CAD build for the part. Positions are in the model's coordinates, mm. A direction names the side the tool comes from. Give positions to 0.01 mm unless a question says otherwise; leave off trailing zeros. Write each loop counter-clockwise with the first axis right and the second up, starting at its lowest first coordinate (ties: lowest second). Pieces come first, ordered by that corner, then holes. Notation, with made-up numbers: (53.25, 12.5) - (95.25, 12.5) arc R29 cw to (95.25, 40.5) - close; hole circle Ø1 at (-4, 59). An arc over 180 degrees is marked (long way). Put each result on its own line as item: value. Start each with the question number.
1. Tool access for faces 1 (the flat face through (46, 9.525, 25)), 2 (the flat face through (29, 9, 7.515)), 3 (the flat face through (-25.03, 22.06, 14.06)): list every direction of +Z, -Z, +X, -X, +Y, -Y with a clear straight run to the whole face (end or side of a thin tool).
2. Cut at A-A on y = 50. List the corners of the cut face in (x, z).
3. Mould opens along Y. For faces 4 (the cylindrical face through (16.81, 30.01, 14.06)), 5 (the cylindrical face through (-21.068, 42.22, 9.623)), 6 (the cylindrical face through (25.477, 0.209, 3.705)), 7 (the cylindrical face through (-15.38, -15.73, 14.06)) say: +Y half, -Y half, draft (parallel to the pull), parting line (faces both ways), or undercut.
4. Drop flat-ended pins along their axis: pin 1 (1 mm diameter, centred on y = 18, z = 3.5, fed in from -X); pin 2 (11.5 mm diameter, centred on x = 46, y = 15, fed in from -Z); pin 3 (4 mm diameter, centred on y = 7, z = 16, fed in from +X); pin 4 (8.5 mm diameter, centred on x = 47, z = 25, fed in from +Y). Give the stop position or say it passes through.
5. Cut at D-D on y = -10.5. List the corners of the cut face in (x, z) (3 decimals), and give its area (3 significant figures).
6. Cut at C-C on x = 21. List the corners of the cut face in (y, z) (3 decimals), and give its area (3 significant figures).
7. Cut at B-B on z = 22. List the corners of the cut face in (x, y) (3 decimals), and give its area (3 significant figures).
8. Wall check: line 1 (Z direction, x = 35, y = 15) (3 decimals); line 2 (X direction, y = 44, z = 14.25); line 3 (Y direction, x = 0, z = 9.5) (1 decimal). Give the ranges that are in metal, low to high.
from build123d import *

# Parameters (mm, degrees)
SKETCH1_R           = 9.525
SKETCH1_R_2         = 7
BOSS_EXTRUDE1_DEPTH = 28.52
CUT_EXTRUDE10_START = -9
CUT_EXTRUDE10_DEPTH = 9
SKETCH5_W           = 38
SKETCH5_H           = 13.49
CUT_EXTRUDE11_DEPTH = 89.917885715
EXTRUDE_THIN4_DEPTH = 9
SKETCH9_W           = 9
SKETCH9_H           = 9
BOSS_EXTRUDE3_DEPTH = 20
SKETCH10_W          = 9
SKETCH10_H          = 10
CUT_EXTRUDE12_DEPTH = 85.459250319


with BuildPart() as part:
    # Sketch1 → Boss-Extrude1 (new body)
    with BuildSketch(Plane.XY):
        with BuildLine():
            Line((-22, 0), (-28.14403802, 44.745229643))
            ThreePointArc((-28.14403802, 44.745229643), (-16.381808273, 59.200012083), (-2.762561842, 46.47967755))
            ThreePointArc((-2.762561842, 46.47967755), (23.974569133, 26.563983764), (57, 22))
            Line((57, 22), (57, 9.525))
            Line((57, 9.525), (35, 9.525))
            ThreePointArc((35, 9.525), (25.475, 0), (35, -9.525))
            Line((35, -9.525), (57, -9.525))
            Line((57, -9.525), (57, -22))
            Line((57, -22), (0, -22))
            ThreePointArc((0, -22), (-15.556349186, -15.556349186), (-22, 0))
        make_face()
        Circle(SKETCH1_R, mode=Mode.SUBTRACT)
        with Locations((-15.512561842, 46.47967755)):
            Circle(SKETCH1_R_2, mode=Mode.SUBTRACT)
    extrude(amount=BOSS_EXTRUDE1_DEPTH)

    # Sketch2 → Cut-Extrude10 (cut)
    with BuildSketch(Plane.XY.offset(28.52).offset(CUT_EXTRUDE10_START)):
        with BuildLine():
            Line((-28.14403802, 44.745229643), (-26.227740449, 30.789395608))
            ThreePointArc((-26.227740449, 30.789395608), (-9.369633943, 28.50012147), (2.563298764, 40.626194538))
            Line((2.563298764, 40.626194538), (-2.762561842, 46.47967755))
            ThreePointArc((-2.762561842, 46.47967755), (-16.381808273, 59.200012083), (-28.14403802, 44.745229643))
        make_face()
    extrude(amount=CUT_EXTRUDE10_DEPTH, mode=Mode.SUBTRACT)

    # Sketch5 → Cut-Extrude11 (cut, through all)
    with BuildSketch(Plane(origin=(0, 40, 0), x_dir=(1, 0, 0), z_dir=(0, 1, 0))):
        with Locations((38, -14.26)):
            Rectangle(SKETCH5_W, SKETCH5_H)
    extrude(amount=-CUT_EXTRUDE11_DEPTH, mode=Mode.SUBTRACT)



with BuildPart() as body_2:
    # Sketch8 → Extrude-Thin4 (new body)
    with BuildSketch(Plane.XY.offset(28.52)):
        Polygon((2.563298764, 40.626194538), (-6.432243018, 40.342948992), (-6.746960292, 50.337995417), (2.248581491, 50.621240963), align=None)
    extrude(amount=-EXTRUDE_THIN4_DEPTH)


with BuildPart() as part_1:
    add(part.part)

    add(body_2.part)  # Boss-Extrude3 merges body 2
    # Sketch9 → Boss-Extrude3 (add)
    with BuildSketch(Plane(origin=(-1.590121568, 50.500370473, 0), x_dir=(0.9995046425001054, 0.0314717273236879, 0), z_dir=(-0.0314717273236879, 0.9995046425001055, 0))):
        with Locations((-0.659394469, -24.02)):
            Rectangle(SKETCH9_W, SKETCH9_H)
    extrude(amount=-BOSS_EXTRUDE3_DEPTH)

    # Sketch10 → Cut-Extrude12 (cut, through all)
    with BuildSketch(Plane(origin=(3.838703059, 0.12087049, 0), x_dir=(0, 0, -1), z_dir=(0.9995046425001055, 0.03147172732368791, 0))):
        with Locations((-24.02, 45.525398608)):
            Rectangle(SKETCH10_W, SKETCH10_H)
    extrude(amount=-CUT_EXTRUDE12_DEPTH, mode=Mode.SUBTRACT)


solid = part_1.part
Report:
1. face 1: +Z, -Z, +X
1. face 2: +X, +Y, -Y
1. face 3: +Z, -Z, -X, -Y
2. outline: (-27.77, 0) - (-21.56, 0) - (-21.56, 19.52) - (-27.77, 19.52) - close; (-9.46, 0) - (-3.26, 0) - (-3.26, 19.52) - (-9.46, 19.52) - close
3. face 4: +Y half
3. face 5: undercut
3. face 6: undercut
3. face 7: -Y half
4. pin 1: stops at x = -24.54
4. pin 2: stops at z = 0
4. pin 3: stops at x = 19
4. pin 4: stops at y = 21.89
5. outline: (-19.333, 0) - (57, 0) - (57, 7.515) - (19, 7.515) - (19, 21.005) - (57, 21.005) - (57, 28.52) - (-19.333, 28.52) - close
5. area: 1,660 mm²
6. outline: (-22, 0) - (27.867, 0) - (27.867, 7.515) - (-22, 7.515) - close; (-22, 21.005) - (27.867, 21.005) - (27.867, 28.52) - (-22, 28.52) - close
6. area: 750 mm²
7. outline: (-26.228, 30.789) - (-22, 0) arc R22 ccw to (0, -22) - (57, -22) - (57, -9.525) - (35, -9.525) arc R9.525 cw to (35, 9.525) - (57, 9.525) - (57, 22) arc R67 cw to (2.563, 40.626) - (-6.432, 40.343) - (-6.118, 30.348) - (-5.44, 30.369) arc R19 cw to start; hole circle Ø19.05 at (0, 0)
7. area: 3,100 mm²
8. line 1: z = 0 to 7.515, 21.005 to 28.52
8. line 2: x = -28.04 to -22.06, -8.97 to -0.66
8. line 3: y = -22 to -9.5, 9.5 to 43.3
